Input: part model. Units: mm. Frame: model coordinates. A direction names the side the tool comes from. Round coordinates to 2 decimals unless told otherwise and drop trailing zeros. Loops run counter-clockwise (first coordinate to the right, second up) from the corner with the lowest first, then second, coordinate; pieces in that order, holes last. Notation, with made-up numbers: (82.5, 80.5) -> (132.5, 80.5) arc R13 ccw to (132.5, 98.5) -> close; hole circle Ø7 at (43, 85). An arc over 180 degrees is marked (long way). One line per question, with ' | ' between items. Start each with the question number.
Q1. Cut plane A-A on z = -7. Return loops of the section in (x, y).
Q2. Mould query, pull axis X, two halves, no side actions, for faces 1 (the face through (55, 5, -5)), 2 (the face through (105, 3, 0)), 3 (the face through (22, 0, 0)). Classes: pulls with the +X half, pulls with the -X half, needs draft (parallel to the pull), parting line crosses it, or undercut.
Q3. Access query for faces 4 (the face through (20, 5, -7)), 5 (the face through (20, 5, 8)), 6 (the face through (90, -1, 0)), 7 (the face through (97, -5, 0)), 8 (the face through (0, 5, 10)). Directions: +Z, -Z, +X, -X, +Y, -Y. A direction counts if a zero-diameter tool reaches every point of the face in a straight line with its end or side. Return the directions, or none.
Q4. Cut plane C-C on x = -1.5. Return loops of the section in (y, z).
Q5. Contact query for flat-ended pins moving along their axis: P1, Ø4, axis at x = 23, z = 6.5, coming from the -Y side; P2, Ø3, axis at x = 46.5, y = 7, coming from the -Z side; P3, Ø5, axis at x = 77.5, y = 6, coming from the +Z side. Output: stop coordinate, or through.
Q6. Material intervals for L1, parallel to X at y = 7.25, z = 7; L2, parallel to Z at x = 51.5, y = 9.25; L3, parallel to Y at x = 86, z = 2.25, sorted ascending.
Q7. Cut plane B-B on y = 2.75. Return loops of the section in (x, z).
Q8. Cut plane D-D on z = 3.5. Return loops of the section in (x, y), and give its area (4 significant figures).
from build123d import *

# Parameters (mm, degrees)
SKETCH1_W           = 70
SKETCH1_H           = 10
SKETCH1_W_2         = 40
SKETCH1_H_2         = 20
BOSS_EXTRUDE1_DEPTH = 10
BOSS_EXTRUDE2_START = 10
BOSS_EXTRUDE2_DEPTH = 15


with BuildPart() as part:
    # Sketch1 → Boss-Extrude1 (new body)
    with BuildSketch(Plane(origin=(0, 0, 0), x_dir=(1, 0, 0), z_dir=(0, 1, 0))):
        with Locations((55, 0)):
            Rectangle(SKETCH1_W, SKETCH1_H)
        Rectangle(SKETCH1_W_2, SKETCH1_H_2)
    extrude(amount=BOSS_EXTRUDE1_DEPTH)

    # Sketch1<3> → Boss-Extrude2 (add)
    with BuildSketch(Plane(origin=(0, 0, 0), x_dir=(1, 0, 0), z_dir=(0, 1, 0)).offset(BOSS_EXTRUDE2_START)):
        Polygon((90, 5), (90, -5), (90, -10), (105, -10), (105, 10), (90, 10), align=None)
    extrude(amount=-BOSS_EXTRUDE2_DEPTH)


solid = part.part
Results:
1) outline: (-20, 0) -> (20, 0) -> (20, 10) -> (-20, 10) -> close; (90, -5) -> (105, -5) -> (105, 10) -> (90, 10) -> close
2) face 1: undercut | face 2: pulls with the +X half | face 3: needs draft
3) face 4: -Z, +Y, -Y | face 5: +Z, +Y, -Y | face 6: -Y | face 7: +Z, -Z, +X, -X, -Y | face 8: +Z, +X, -X, +Y, -Y
4) outline: (0, -10) -> (10, -10) -> (10, 10) -> (0, 10) -> close
5) P1: y = 0 | P2: z = -5 | P3: z = 5
6) L1: -20 to 20, 90 to 105 | L2: -5 to 5 | L3: 0 to 10
7) outline: (-20, -10) -> (20, -10) -> (20, -5) -> (90, -5) -> (90, -10) -> (105, -10) -> (105, 10) -> (90, 10) -> (90, 5) -> (20, 5) -> (20, 10) -> (-20, 10) -> close
8) outline: (-20, 0) -> (90, 0) -> (90, -5) -> (105, -5) -> (105, 10) -> (-20, 10) -> close | area: 1,325 mm^2
